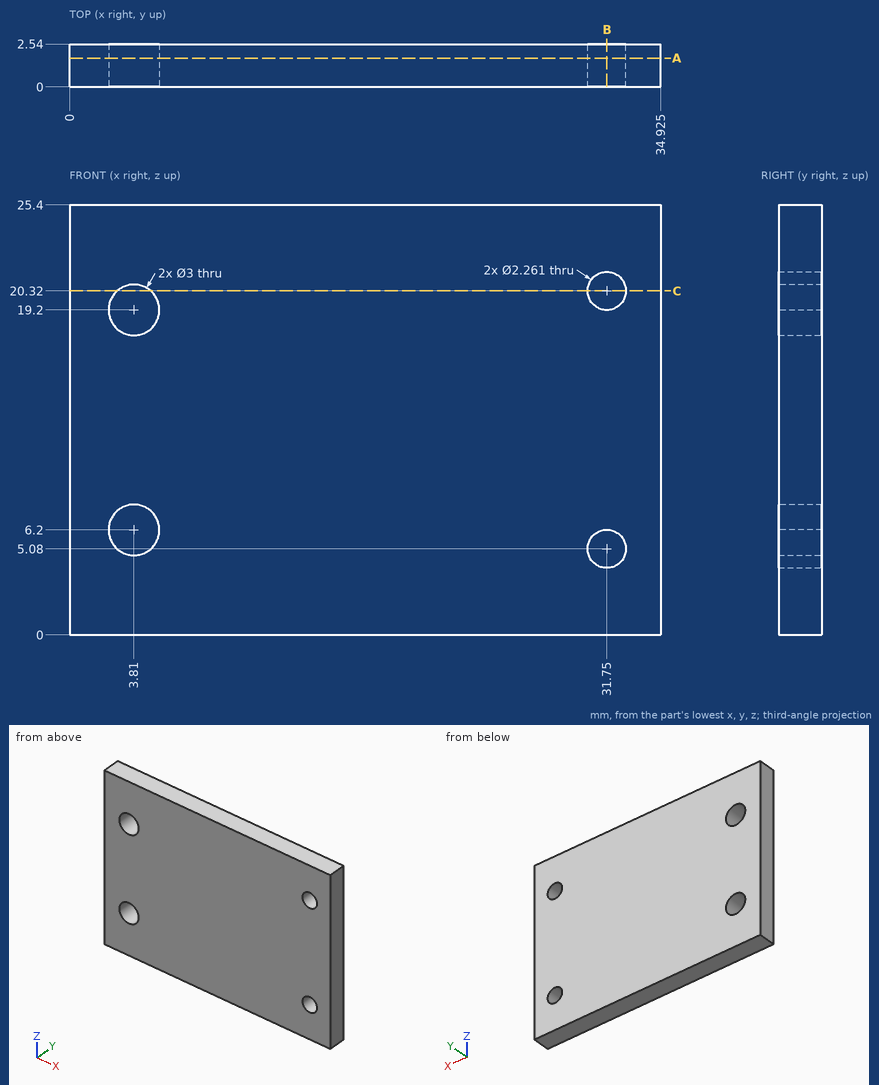
For this review, use the dimensioned drawing (mm, ordinates from the lowest corner) and the shaded views. Round coordinates to 2 decimals unless told otherwise and drop trailing zeros. Order: outer loops, then holes, each group sorted by start corner. A loop starts at its lowest first (then second) coordinate and runs counter-clockwise, first axis right, second up.
1) Consider section C-C (z = 20.32). State the section outline as (x, y) points (1 decimal).
The answers:
outline: (0, 0) - (2.8, 0) - (2.8, 2.5) - (0, 2.5) - close; (4.8, 0) - (30.6, 0) - (30.6, 2.5) - (4.8, 2.5) - close; (32.9, 0) - (34.9, 0) - (34.9, 2.5) - (32.9, 2.5) - close
2) Clearance check with a flat-ended pin moving along its axis: pin 1 Ø1.8 at (x, z) = (31.75, 5.08) entering from +Y. State where the tip first meets the part, or that it passes through.
The answers:
pin 1: passes through
3) For L1, parallel to X at y = 0.3, z = 5.75 (1 decimal); L2, parallel to X at y = 1.55, z = 19.5 (1 decimal); L3, parallel to X at y = 1.5, z = 18.5 (1 decimal), list the stretches that pass through material, from the lowest coordinate up.
The answers:
L1: x = 0 to 2.4, 5.2 to 30.8, 32.7 to 34.9
L2: x = 0 to 2.3, 5.3 to 31, 32.5 to 34.9
L3: x = 0 to 2.5, 5.1 to 34.9
4) Consider section A-A (y = 1.7). Count the separate pieces of the cut face and the enclosed holes in it, plus the area to 3 significant figures.
The answers:
separate pieces: 1
enclosed holes: 4
area: 865 mm2
5) Consider section B-B (x = 31.75). State the section outline as (y, z) points.
The answers:
outline: (0, 0) - (2.54, 0) - (2.54, 3.95) - (0, 3.95) - close; (0, 6.21) - (2.54, 6.21) - (2.54, 19.19) - (0, 19.19) - close; (0, 21.45) - (2.54, 21.45) - (2.54, 25.4) - (0, 25.4) - close
